from build123d import *

# Parameters (mm, degrees)
EXTRUDE_START                = -9
EXTRUDE_1_DEPTH              = 18
SKETCH_5_R                   = 1
CUT_EXTRUDE_1_DEPTH          = 3
HOLE_WIZARD_M3_1_D           = 2.5
HOLE_WIZARD_M3_1_DEPTH       = 4
HOLE_WIZARD_M3_1_CSINK_D     = 2.55
HOLE_WIZARD_M3_1_CSINK_ANGLE = 90
HOLE_WIZARD_M3_1_TIP         = 0.751075774


# Read off the part's stored shape, not the designer's step: 凸台-拉伸1
with BuildPart() as part:
    # 凸台-拉伸1 outline → 凸台-拉伸1 (new body)
    with BuildSketch(Plane.XY.offset(EXTRUDE_START)):
        Polygon((67.226055932, -71.547534757), (68.220489275, -69.812281944), (50.867961141, -59.867948514), (49.873527798, -61.603201327), (49.005901391, -61.105984655), (49.503118063, -60.238358249), (48.635491656, -59.741141577), (40.18280824, -74.490790491), (61.005842001, -86.423990607), (69.458525416, -71.674341694), (68.59089901, -71.177125022), (68.093682338, -72.044751429), align=None)
    extrude(amount=EXTRUDE_1_DEPTH)

    # 草图5 → 切除-拉伸1 (cut)
    with BuildSketch(Plane(origin=(-13.251129944, -23.122777084, 0), x_dir=(0.8676264066772513, -0.49721667151888715, 0), z_dir=(0.49721667151888715, 0.8676264066772513, 0))):
        with Locations(Location((83.90172843, 5, 0), (0, 0, 180))):
            Circle(SKETCH_5_R)
        with Locations(Location((83.90172843, -5, 0), (0, 0, 180))):
            Circle(SKETCH_5_R)
    extrude(amount=-CUT_EXTRUDE_1_DEPTH, mode=Mode.SUBTRACT)

    # M3 螺纹孔的螺纹孔钻头1
    with Locations(Plane(origin=(-13.251129944, -23.122777084, 0), x_dir=(0.8676264066772513, -0.49721667151888715, 0), z_dir=(0.49721667151888715, 0.8676264066772513, 0))):
        with Locations((83.90172843, 5), (83.90172843, -5)):
            CounterSinkHole(HOLE_WIZARD_M3_1_D / 2, HOLE_WIZARD_M3_1_CSINK_D / 2, depth=HOLE_WIZARD_M3_1_DEPTH, counter_sink_angle=HOLE_WIZARD_M3_1_CSINK_ANGLE)
            with Locations((0, 0, -(HOLE_WIZARD_M3_1_DEPTH + HOLE_WIZARD_M3_1_TIP / 2))):  # 118° drill point
                Cone(0, HOLE_WIZARD_M3_1_D / 2, HOLE_WIZARD_M3_1_TIP, mode=Mode.SUBTRACT)


solid = part.part
CAD build for the part. Positions are in the model's coordinates, mm. A direction names the side the tool comes from. Coordinates: 2 decimals unless noted, no trailing zeros. Loops run counter-clockwise (first coordinate to the right, second up) from the corner with the lowest first, then second, coordinate; pieces in that order, holes last. Notation, with made-up numbers: (70, 30.25) - (80, 30.25) arc R29 cw to (80, 57.25) - close; hole circle Ø4 at (2.25, -8.5). An arc over 180 degrees is marked (long way). Write item = value, one per line. Start each with the question number.
Q1. Drill centre lines: L1, parallel to X at y = -65.5, z = -5.5; L2, parallel to Y at x = 67, z = 7.25; L3, parallel to X at y = -76.75, z = 1.25. Where is each one in solid material? Low to high.
Q2. Which spindle directions (+Z, -Z, +X, -X, +Y, -Y) get a long thin tool onto all of the face, cutting with end or side? Do faces 4 (the flat face through (49.075, -59.993, -0.126)), 5 (the flat face through (55, -73, 9)), 6 (the flat face through (67.67, -71.8, -0.13)), 7 (the conical face through (57.06, -68.74, 4.99)). Say none if no direction does.
Q3. Flat gauge pins, fed straight in: pin 1 Ø4 at (y, z) = (-65, -3) entering from -X; pin 2 Ø4 at (x, z) = (44.5, 0) entering from -Y; pin 3 Ø8 at (y, z) = (-79.5, 5) entering from +X. Where does each tip first touch, or does it go through?
Q4. Cut at A-A, the plane z = -7.5. List the corners of the cut face in (x, y).
Q5. Pull direction Z, two halves, no side cores. Call faces 1 (the flat face through (55, -73, -9)), 2 (the conical face through (57.06, -68.74, -5.01)), 3 (the flat face through (65.173, -79.152, -0.126)): pulls with the +Z half, pulls with the -Z half, needs draft (parallel to the pull), parting line crosses it, or undercut.
Q6. Cut at C-C, the plane y = -79. List the corners of the cut face in (x, z), then the cut area to 3 significant figures.
Q7. Cut at B-B, the plane x = 45.5. List the corners of the cut face in (y, z), then the cut area to 3 significant figures.
Computed:
q1.L1 = 45.34 to 57.85, 60.49 to 60.7
q1.L2 = -75.96 to -69.11
q1.L3 = 44.13 to 66.55
q2.face_4 = +Z, -Z, +Y
q2.face_5 = +Z, +X, -X, +Y, -Y
q2.face_6 = +Z, -Z
q2.face_7 = none
q3.pin_1 = 44.48
q3.pin_2 = -78.11
q3.pin_3 = 67.27
q4.outline = (40.18, -74.49) - (61.01, -86.42) - (69.46, -71.67) - (68.59, -71.18) - (68.09, -72.04) - (67.23, -71.55) - (68.22, -69.81) - (50.87, -59.87) - (49.87, -61.6) - (49.01, -61.11) - (49.5, -60.24) - (48.64, -59.74) - close
q5.face_1 = pulls with the -Z half
q5.face_2 = undercut
q5.face_3 = needs draft
q6.outline = (48.05, -9) - (65.26, -9) - (65.26, 9) - (48.05, 9) - close
q6.area = 310 mm²
q7.outline = (-77.54, -9) - (-65.21, -9) - (-65.21, 9) - (-77.54, 9) - close
q7.area = 222 mm²
